The listing builds one solid part. Answer for the finished solid, in the listing's coordinates (mm). A direction names the side the tool comes from. Round coordinates to 2 decimals unless told otherwise and drop trailing zeros. Loops run counter-clockwise (first coordinate to the right, second up) from the corner with the lowest first, then second, coordinate; pieces in that order, holes last. Notation, with made-up numbers: (53.25, 65.25) -> (82.25, 65.25) arc R12 ccw to (82.25, 80.25) -> close; hole circle Ø7 at (-33, 88.25). An arc over 180 degrees is marked (long way). Use a Markdown table: item, result. Add a question column.
Q1. Section C-C on y = 75.5 is taken. Give the vertices of the cut face in (x, z).
Q2. Which of the six approach directions +Z, -Z, +X, -X, +Y, -Y give full straight-line access (tool end or side, diameter ignored) to faces 1 (the flat face through (42, 56, 5)), 2 (the cylindrical face through (5.795, 101.327, 3.274)), 3 (the cylindrical face through (1.5, 93.93, 2.46)), 4 (the flat face through (57, 60, 3)), 5 (the cylindrical face through (58, 109, 3))?
Q3. Given pin 1 Ø5 at (x, y) = (53.5, 6) entering from +Z; pin 2 Ø2 at (y, z) = (27.5, 3.5) entering from -X; pin 3 Ø1 at (x, z) = (57.5, 2.5) entering from +Y, each flat-ended and moving along its own axis, determine where each tip first touches the part or whether it passes through.
Q4. Section A-A on x = 53.5 is taken. Give the vertices of the cut face in (y, z).
Q5. Consider line 1 (Y direction, x = 6.5, z = 4); line 2 (Y direction, x = 53.5, z = 3.05); line 3 (Y direction, x = 10, z = 4.6). Determine where each line is inside the solid, lowest interval first.
Q6. Section B-B on x = 6.5 is taken. Give the vertices of the cut face in (y, z).
Q7. Section D-D on x = 22.5 is taken. Give the vertices of the cut face in (y, z).
from build123d import *
from build123d.topology import SkipClean

# Parameters (mm, degrees)
BOSS_EXTRUDE1_DEPTH = 5
SKETCH3_R           = 2.1
CUT_EXTRUDE1_DEPTH  = 10
BOSS_EXTRUDE2_DEPTH = 5
SKETCH4_3_R         = 2.1
CUT_EXTRUDE2_DEPTH  = 5
FILLET1_R           = 5
SKETCH5_W           = 25
SKETCH5_H           = 75
SKETCH5_W_2         = 15.371996706
SKETCH5_H_2         = 32.5
CUT_EXTRUDE3_DEPTH  = 5
FILLET2_R           = 5
SKETCH6_R           = 3.25
CUT_EXTRUDE4_DEPTH  = 3.5


with BuildPart() as part:
    # Sketch1 → Boss-Extrude1 (new body)
    with BuildSketch(Plane.XY):
        Polygon((60, 40), (60, 110), (0, 110), (0, 0), (60, 0), align=None)
    extrude(amount=BOSS_EXTRUDE1_DEPTH)

    # Sketch3 → Cut-Extrude1 (cut)
    with BuildSketch(Plane.XY.offset(5)):
        with Locations((6.5, 5.5)):
            Circle(SKETCH3_R)
        with Locations((53.5, 5.5)):
            Circle(SKETCH3_R)
        with Locations(Location((53.5, 104.5, 0), (0, 0, 180))):
            Circle(SKETCH3_R)
        with Locations(Location((6.5, 104.5, 0), (0, 0, 180))):
            Circle(SKETCH3_R)
    extrude(amount=-CUT_EXTRUDE1_DEPTH, mode=Mode.SUBTRACT)

    # Sketch4 → Boss-Extrude2 (add)
    with BuildSketch(Plane.XY.offset(5)):
        with BuildLine():
            Line((70, 60), (60, 60))
            Line((60, 60), (60, 49.039607805))
            ThreePointArc((60, 49.039607805), (61.79614814, 48.652271164), (62.6, 47))
            ThreePointArc((62.6, 47), (61.79614814, 45.347728836), (60, 44.960392195))
            Line((60, 44.960392195), (60, 32.039607805))
            ThreePointArc((60, 32.039607805), (61.79614814, 31.652271164), (62.6, 30))
            ThreePointArc((62.6, 30), (61.79614814, 28.347728836), (60, 27.960392195))
            Line((60, 27.960392195), (60, 10))
            Line((60, 10), (70, 10))
            Line((70, 10), (70, 60))
        make_face()
    extrude(amount=-BOSS_EXTRUDE2_DEPTH)

    # Sketch4<3> → Cut-Extrude2 (cut)
    with SkipClean():  # the faces are left unmerged after this step: merging them gives an invalid solid
        with BuildSketch(Plane.XY.offset(5)):
            with Locations((60.5, 30)):
                Circle(SKETCH4_3_R)
            with Locations((44.5, 30)):
                Circle(SKETCH4_3_R)
            with Locations((44.5, 47)):
                Circle(SKETCH4_3_R)
            with Locations((60.5, 47)):
                Circle(SKETCH4_3_R)
        extrude(amount=-CUT_EXTRUDE2_DEPTH, mode=Mode.SUBTRACT)

    # Fillet1
    fillet1_edges = [part.edges().sort_by_distance(p)[0] for p in [
        (0, 110, 2.5),
        (0, 0, 2.5),
    ]]
    fillet(fillet1_edges, radius=FILLET1_R)

    # Sketch5 → Cut-Extrude3 (cut)
    with BuildSketch(Plane.XY.offset(5)):
        with Locations((12.5, 55)):
            Rectangle(SKETCH5_W, SKETCH5_H)
        with Locations((52.314001647, 76.25)):
            Rectangle(SKETCH5_W_2, SKETCH5_H_2)
    extrude(amount=-CUT_EXTRUDE3_DEPTH, mode=Mode.SUBTRACT)

    # Fillet2
    fillet2_edges = [part.edges().sort_by_distance(p)[0] for p in [
        (60, 0, 2.5),
        (60, 10, 2.5),
        (70, 10, 2.5),
        (70, 60, 2.5),
        (60, 92.5, 2.5),
        (60, 110, 2.5),
        (44.628003294, 92.5, 2.5),
        (44.628003294, 60, 2.5),
        (0, 17.5, 2.5),
        (25, 17.5, 2.5),
        (25, 92.5, 2.5),
        (0, 92.5, 2.5),
    ]]
    fillet(fillet2_edges, radius=FILLET2_R - 0.0001)  # a hair under: the kernel refuses the full size

    # Sketch6 → Cut-Extrude4 (cut)
    with BuildSketch(Plane.XY.offset(5)):
        with Locations((44.5, 47)):
            Circle(SKETCH6_R)
        with Locations((60.5, 47)):
            Circle(SKETCH6_R)
        with Locations((60.5, 30)):
            Circle(SKETCH6_R)
        with Locations((44.5, 30)):
            Circle(SKETCH6_R)
        with Locations((53.5, 5.5)):
            Circle(SKETCH6_R)
        with Locations((6.5, 5.5)):
            Circle(SKETCH6_R)
        with Locations((6.5, 104.5)):
            Circle(SKETCH6_R)
        with Locations((53.5, 104.5)):
            Circle(SKETCH6_R)
    extrude(amount=-CUT_EXTRUDE4_DEPTH, mode=Mode.SUBTRACT)


solid = part.part
Checked values:
| question | item | result |
|---|---|---|
| 1 | outline | (25, 0) -> (44.63, 0) -> (44.63, 5) -> (25, 5) -> close |
| 2 | face 1 | +Z, +X, -X, +Y, -Y |
| 2 | face 2 | +Z |
| 2 | face 3 | +Z, -Z, -X |
| 2 | face 4 | +Z, -Z, +X |
| 2 | face 5 | +Z, -Z, +X, +Y |
| 3 | pin 1 | stops at z = 1.5 |
| 3 | pin 2 | stops at x = 25 |
| 3 | pin 3 | stops at y = 109.58 |
| 4 | outline | (0, 0) -> (3.4, 0) -> (3.4, 1.5) -> (2.25, 1.5) -> (2.25, 5) -> (0, 5) -> close; (7.6, 0) -> (60, 0) -> (60, 5) -> (8.75, 5) -> (8.75, 1.5) -> (7.6, 1.5) -> close; (92.5, 0) -> (102.4, 0) -> (102.4, 1.5) -> (101.25, 1.5) -> (101.25, 5) -> (92.5, 5) -> close; (106.6, 0) -> (110, 0) -> (110, 5) -> (107.75, 5) -> (107.75, 1.5) -> (106.6, 1.5) -> close |
| 5 | line 1 | y = 0 to 2.25, 8.75 to 17.5, 92.5 to 101.25, 107.75 to 110 |
| 5 | line 2 | y = 0 to 2.25, 8.75 to 60, 92.5 to 101.25, 107.75 to 110 |
| 5 | line 3 | y = 0 to 17.5, 92.5 to 110 |
| 6 | outline | (0, 0) -> (3.4, 0) -> (3.4, 1.5) -> (2.25, 1.5) -> (2.25, 5) -> (0, 5) -> close; (7.6, 0) -> (17.5, 0) -> (17.5, 5) -> (8.75, 5) -> (8.75, 1.5) -> (7.6, 1.5) -> close; (92.5, 0) -> (102.4, 0) -> (102.4, 1.5) -> (101.25, 1.5) -> (101.25, 5) -> (92.5, 5) -> close; (106.6, 0) -> (110, 0) -> (110, 5) -> (107.75, 5) -> (107.75, 1.5) -> (106.6, 1.5) -> close |
| 7 | outline | (0, 0) -> (18.17, 0) -> (18.17, 5) -> (0, 5) -> close; (91.83, 0) -> (110, 0) -> (110, 5) -> (91.83, 5) -> close |
